Source: CAD feature listing. Evaluate the final solid. Frame: model axes, mm. Give positions to 0.01 mm unless a question says otherwise; leave off trailing zeros. Loops run counter-clockwise (first coordinate to the right, second up) from the corner with the lowest first, then second, coordinate; pieces in that order, holes last.
```python
from build123d import *

# Parameters (mm, degrees)
SKETCH_1_R      = 10
SKETCH_1_R_2    = 2
SKETCH_1_R_3    = 5.5
EXTRUDE_1_DEPTH = 3


with BuildPart() as part:
    # 草图1 → 凸台-拉伸1 (new body)
    with BuildSketch(Plane.XY):
        with BuildLine():
            Line((224.953360513, -85.216557036), (224.953360513, -86.716557036))
            Line((224.953360513, -86.716557036), (227.553360513, -86.716557036))
            Line((227.553360513, -86.716557036), (227.553360513, -85.216557036))
            Line((227.553360513, -85.216557036), (230.553360513, -85.216557036))
            Line((230.553360513, -85.216557036), (230.553360513, -82.216557036))
            Line((230.553360513, -82.216557036), (227.553360513, -82.216557036))
            Line((227.553360513, -82.216557036), (227.553360513, -80.716557036))
            Line((227.553360513, -80.716557036), (224.953360513, -80.716557036))
            Line((224.953360513, -80.716557036), (224.953360513, -82.216557036))
            Line((224.953360513, -82.216557036), (222.453360513, -82.216557036))
            Line((222.453360513, -82.216557036), (222.453360513, 246.962931603))
            Line((222.453360513, 246.962931603), (224.953360513, 246.962931603))
            Line((224.953360513, 246.962931603), (224.953360513, 245.462931603))
            Line((224.953360513, 245.462931603), (227.553360513, 245.462931603))
            Line((227.553360513, 245.462931603), (227.553360513, 246.962931603))
            Line((227.553360513, 246.962931603), (230.553360513, 246.962931603))
            Line((230.553360513, 246.962931603), (230.553360513, 249.962931603))
            Line((230.553360513, 249.962931603), (227.553360513, 249.962931603))
            Line((227.553360513, 249.962931603), (227.553360513, 251.462931603))
            Line((227.553360513, 251.462931603), (224.953360513, 251.462931603))
            Line((224.953360513, 251.462931603), (224.953360513, 249.962931603))
            Line((224.953360513, 249.962931603), (222.453360513, 249.962931603))
            Line((222.453360513, 249.962931603), (222.453360513, 275.962931603))
            ThreePointArc((222.453360513, 275.962931603), (249.953360513, 303.462931603), (277.453360513, 275.962931603))
            Line((277.453360513, 275.962931603), (277.453360513, 249.962931603))
            Line((277.453360513, 249.962931603), (274.953360513, 249.962931603))
            Line((274.953360513, 249.962931603), (274.953360513, 251.462931603))
            Line((274.953360513, 251.462931603), (272.353360513, 251.462931603))
            Line((272.353360513, 251.462931603), (272.353360513, 249.962931603))
            Line((272.353360513, 249.962931603), (269.353360513, 249.962931603))
            Line((269.353360513, 249.962931603), (269.353360513, 246.962931603))
            Line((269.353360513, 246.962931603), (272.353360513, 246.962931603))
            Line((272.353360513, 246.962931603), (272.353360513, 245.462931603))
            Line((272.353360513, 245.462931603), (274.953360513, 245.462931603))
            Line((274.953360513, 245.462931603), (274.953360513, 246.962931603))
            Line((274.953360513, 246.962931603), (277.453360513, 246.962931603))
            Line((277.453360513, 246.962931603), (277.453360513, 137.142420241))
            Line((277.453360513, 137.142420241), (274.953360513, 137.142420241))
            Line((274.953360513, 137.142420241), (274.953360513, 138.642420241))
            Line((274.953360513, 138.642420241), (272.353360513, 138.642420241))
            Line((272.353360513, 138.642420241), (272.353360513, 137.142420241))
            Line((272.353360513, 137.142420241), (269.353360513, 137.142420241))
            Line((269.353360513, 137.142420241), (269.353360513, 134.142420241))
            Line((269.353360513, 134.142420241), (272.353360513, 134.142420241))
            Line((272.353360513, 134.142420241), (272.353360513, 132.642420241))
            Line((272.353360513, 132.642420241), (274.953360513, 132.642420241))
            Line((274.953360513, 132.642420241), (274.953360513, 134.142420241))
            Line((274.953360513, 134.142420241), (277.453360513, 134.142420241))
            Line((277.453360513, 134.142420241), (277.453360513, -195.037068397))
            Line((277.453360513, -195.037068397), (274.953360513, -195.037068397))
            Line((274.953360513, -195.037068397), (274.953360513, -193.537068397))
            Line((274.953360513, -193.537068397), (272.353360513, -193.537068397))
            Line((272.353360513, -193.537068397), (272.353360513, -195.037068397))
            Line((272.353360513, -195.037068397), (269.353360513, -195.037068397))
            Line((269.353360513, -195.037068397), (269.353360513, -198.037068397))
            Line((269.353360513, -198.037068397), (272.353360513, -198.037068397))
            Line((272.353360513, -198.037068397), (272.353360513, -199.537068397))
            Line((272.353360513, -199.537068397), (274.953360513, -199.537068397))
            Line((274.953360513, -199.537068397), (274.953360513, -198.037068397))
            Line((274.953360513, -198.037068397), (277.453360513, -198.037068397))
            Line((277.453360513, -198.037068397), (277.453360513, -224.037068397))
            ThreePointArc((277.453360513, -224.037068397), (249.953360513, -251.537068397), (222.453360513, -224.037068397))
            Line((222.453360513, -224.037068397), (222.453360513, -198.037068397))
            Line((222.453360513, -198.037068397), (224.953360513, -198.037068397))
            Line((224.953360513, -198.037068397), (224.953360513, -199.537068397))
            Line((224.953360513, -199.537068397), (227.553360513, -199.537068397))
            Line((227.553360513, -199.537068397), (227.553360513, -198.037068397))
            Line((227.553360513, -198.037068397), (230.553360513, -198.037068397))
            Line((230.553360513, -198.037068397), (230.553360513, -195.037068397))
            Line((230.553360513, -195.037068397), (227.553360513, -195.037068397))
            Line((227.553360513, -195.037068397), (227.553360513, -193.537068397))
            Line((227.553360513, -193.537068397), (224.953360513, -193.537068397))
            Line((224.953360513, -193.537068397), (224.953360513, -195.037068397))
            Line((224.953360513, -195.037068397), (222.453360513, -195.037068397))
            Line((222.453360513, -195.037068397), (222.453360513, -85.216557036))
            Line((222.453360513, -85.216557036), (224.953360513, -85.216557036))
        make_face()
        with Locations((249.953360513, 275.962931603)):
            Circle(SKETCH_1_R, mode=Mode.SUBTRACT)
        with Locations((230.953360513, 275.962931603)):
            Circle(SKETCH_1_R_2, mode=Mode.SUBTRACT)
        with Locations((236.518331671, 289.397960445)):
            Circle(SKETCH_1_R_2, mode=Mode.SUBTRACT)
        with Locations((249.953360513, 294.962931603)):
            Circle(SKETCH_1_R_2, mode=Mode.SUBTRACT)
        with Locations((263.388389356, 289.397960445)):
            Circle(SKETCH_1_R_2, mode=Mode.SUBTRACT)
        with Locations((268.953360513, 275.962931603)):
            Circle(SKETCH_1_R_2, mode=Mode.SUBTRACT)
        with Locations((263.388389356, 262.52790276)):
            Circle(SKETCH_1_R_2, mode=Mode.SUBTRACT)
        with Locations((249.953360513, 256.962931603)):
            Circle(SKETCH_1_R_2, mode=Mode.SUBTRACT)
        with Locations((236.518331671, 262.52790276)):
            Circle(SKETCH_1_R_2, mode=Mode.SUBTRACT)
        with Locations((249.953360513, -224.037068397)):
            Circle(SKETCH_1_R_3, mode=Mode.SUBTRACT)
        with BuildLine():
            Line((233.453360513, 232.962931603), (265.776162867, 232.962931603))
            ThreePointArc((265.776162867, 232.962931603), (268.007619579, 231.968075224), (268.759090329, 229.643332232))
            Line((268.759090329, 229.643332232), (236.436287975, -72.036156407))
            ThreePointArc((236.436287975, -72.036156407), (233.293332993, -74.712285861), (230.453360513, -71.716557036))
            Line((230.453360513, -71.716557036), (230.453360513, 229.962931603))
            ThreePointArc((230.453360513, 229.962931603), (231.33204017, 232.084251946), (233.453360513, 232.962931603))
        make_face(mode=Mode.SUBTRACT)
        with BuildLine():
            Line((269.453360513, 123.642420241), (269.453360513, -178.037068397))
            ThreePointArc((269.453360513, -178.037068397), (268.574680857, -180.158388741), (266.453360513, -181.037068397))
            Line((266.453360513, -181.037068397), (234.130558159, -181.037068397))
            ThreePointArc((234.130558159, -181.037068397), (231.899101447, -180.042212019), (231.147630697, -177.717469026))
            Line((231.147630697, -177.717469026), (263.470433052, 123.962019612))
            ThreePointArc((263.470433052, 123.962019612), (266.613388034, 126.638149066), (269.453360513, 123.642420241))
        make_face(mode=Mode.SUBTRACT)
    extrude(amount=EXTRUDE_1_DEPTH)


solid = part.part
```
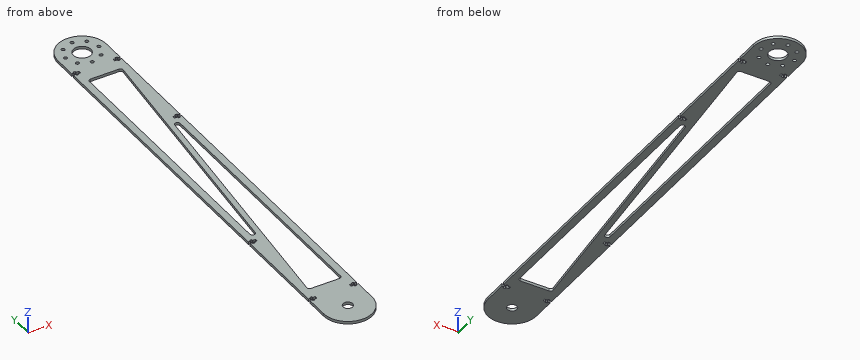
(1) Ray query, line 1 along X through (y, z) = (245.5, 2); line 2 along X through (y, z) = (63.5, 1.1); line 3 along Y through (x, z) = (269, 0.8). Return the intervals inside material, ascending.
A:
line 1: x = 222.45 to 224.95, 227.55 to 272.35, 274.95 to 277.45
line 2: x = 222.45 to 230.45, 250.96 to 256.99, 269.45 to 277.45
line 3: y = -243.87 to -179.62, 125.23 to 273.96, 277.96 to 295.8
(2) Section A-A, the plane y = -119.5. Return the cut outline in (x, z).
A:
outline: (222.45, 0) - (237.39, 0) - (237.39, 3) - (222.45, 3) - close; (269.45, 0) - (277.45, 0) - (277.45, 3) - (269.45, 3) - close
(3) Section B-B, the plane y = -2. Return the cut outline in (x, z).
A:
outline: (222.45, 0) - (230.45, 0) - (230.45, 3) - (222.45, 3) - close; (243.94, 0) - (249.97, 0) - (249.97, 3) - (243.94, 3) - close; (269.45, 0) - (277.45, 0) - (277.45, 3) - (269.45, 3) - close
(4) Section C-C, the plane z = 0.65. Count the separate pieces of the cut face and the enclosed holes in it, then the cut area to 3 significant figures.
A:
separate pieces: 1
enclosed holes: 12
area: 15,500 mm2
(5) Section D-D, the plane y = 172.5. Return the cut outline in (x, z).
A:
outline: (222.45, 0) - (230.45, 0) - (230.45, 3) - (222.45, 3) - close; (262.64, 0) - (277.45, 0) - (277.45, 3) - (262.64, 3) - close
(6) First-contact query: pin 1 (0.9 mm diameter, centred on y = 249, z = 2, fed in from -X); pin 2 (1.3 mm diameter, centred on x = 226.5, z = 1.5, fed in from -Y); pin 3 (1.5 mm diameter, centred on x = 228.5, z = 1.5, fed in from +Y). Flat tips, straight axial feed; report the tip coordinate or a pass-through.
A:
pin 1: stops at x = 230.55
pin 2: stops at y = -239.41
pin 3: stops at y = 294.06
